Design review of the part built by this model. Coordinates are the model's own, in mm. A direction names the side the tool comes from. Give positions to 0.01 mm unless a question says otherwise; leave off trailing zeros. Loops run counter-clockwise (first coordinate to the right, second up) from the corner with the lowest first, then second, coordinate; pieces in that order, holes last.
from build123d import *

# Parameters (mm, degrees)
F0_R     = 22.225
F1_DEPTH = 2.54
F2_R     = 3.81
F2_W     = 3.2512
F2_H     = 3.2512
F3_DEPTH = 19.05


with BuildPart() as f1:
    # F0 (on Front) → F1 (new body)
    with BuildSketch(Plane.XZ):
        with Locations((-29.829953, 27.933979)):
            Circle(F0_R)
    extrude(amount=F1_DEPTH)

    # F2 (on face) → F3 (join)
    with BuildSketch(Plane.XZ.offset(2.54)):
        with Locations((-29.829953, 27.933979)):
            Circle(F2_R)
        with Locations((-29.829953, 27.952339)):
            Rectangle(F2_W, F2_H, mode=Mode.SUBTRACT)
    extrude(amount=F3_DEPTH)


solid = f1.part
Q1. Draft analysis for pull direction X (two halves, no side actions). For faces 1 (the face through (-28.204, -12, 28)), 2 (the face through (-28, -21.59, 28)), 3 (the face through (-26.196, -11.932, 29.078)), state which applies: pulls with the +X half, pulls with the -X half, needs draft (parallel to the pull), parting line crosses it, or undercut.
Results:
face 1: undercut
face 2: needs draft
face 3: parting line crosses it
Q2. Tool access review of faces 4 (the face through (-9.3, -1.25, 19.42)), 5 (the face through (-30, -2.54, 28)): name each direction out of +Z, -Z, +X, -X, +Y, -Y from which nothing blocks a thin tool from reaching the whole face with its end or side.
Results:
face 4: +Y, -Y
face 5: -Y
Q3. Take a section at A-A (x = -29.5). Give the boundary of the cut face in (y, z), plus the area to 3 significant figures.
Results:
outline: (-21.59, 24.14) - (-2.54, 24.14) - (-2.54, 5.71) - (0, 5.71) - (0, 50.16) - (-2.54, 50.16) - (-2.54, 31.73) - (-21.59, 31.73) - (-21.59, 29.58) - (-2.54, 29.58) - (-2.54, 26.33) - (-21.59, 26.33) - close
area: 196 mm2
Q4. Take a section at B-B (y = -15.75). Give the boundary of the cut face in (x, z), plus the area to 3 significant figures.
Results:
outline: circle Ø7.62 at (-29.83, 27.93); hole (-31.46, 26.33) - (-28.2, 26.33) - (-28.2, 29.58) - (-31.46, 29.58) - close
area: 35.0 mm2
Q5. Insertion check: pin 1 (13.5 mm diameter, centred on x = -27, z = 37, fed in from -Y); pin 2 (3.5 mm diameter, centred on y = -8.5, z = 28, fed in from -X); pin 3 (1 mm diameter, centred on y = -6.5, z = 33.5, fed in from -X); pin 4 (8 mm diameter, centred on x = -33, z = 41.5, fed in from -Y). Each pin has a flat end and moves straight along its axis. Give the tip position at first contact, or say it passes through.
Results:
pin 1: stops at y = -21.59
pin 2: stops at x = -33.64
pin 3: passes through
pin 4: stops at y = -2.54
Q6. Take a section at D-D (x = -45.5). Give the boundary of the cut face in (y, z).
Results:
outline: (-2.54, 12.17) - (0, 12.17) - (0, 43.69) - (-2.54, 43.69) - close
Q7. Take a section at C-C (z = 41). Give the boundary of the cut face in (x, y).
Results:
outline: (-47.81, -2.54) - (-11.85, -2.54) - (-11.85, 0) - (-47.81, 0) - close
Q8. Wall thickness on line 1 (X direction, y = -9.25, z = 28.5); line 2 (Y direction, x = -37.5, z = 14); line 3 (X direction, y = -19.25, z = 29.5): over which ranges is each line inside the solid? List them lowest first.
Results:
line 1: x = -33.6 to -31.46, -28.2 to -26.06
line 2: y = -2.54 to 0
line 3: x = -33.3 to -31.46, -28.2 to -26.36
